Autodesk Inventor part; units mm, degrees
ref_plane "Work Plane1" through (0, 485, 0) normal (0, -1, 0) x (1, 0, 0)
ref_plane "YZ Plane" through (0, 0, 0) normal (1, 0, 0) x (0, 1, 0)
ref_plane "XZ Plane" through (0, 0, 0) normal (0, 1, 0) x (-1, 0, 0)
sketch "Sketch1" plane through (0, 0, 0) normal (0, 1, 0) x (-1, 0, 0)
  line L0 (-12, 14) -> (12, 14) construction
  line L1 (14, 12) -> (14, -12) construction
  line L2 (12, -14) -> (-12, -14) construction
  line L3 (-14, -12) -> (-14, 12) construction
  line L4 (-14, 14) -> (14, -14) construction
  line L5 (14, 14) -> (-14, -14) construction
  arc A0 (14, 12) -> (12, 14) centre (12, 12) ccw construction
  arc A1 (12, -14) -> (14, -12) centre (12, -12) ccw construction
  arc A2 (-14, -12) -> (-12, -14) centre (-12, -12) ccw construction
  arc A3 (-12, 14) -> (-14, 12) centre (-12, 12) ccw construction
  line L6 (-12, -15) -> (12, -15)
  arc A4 (12, -15) -> (15, -12) centre (12, -12) ccw
  line L7 (15, -12) -> (15, 12)
  arc A5 (15, 12) -> (12, 15) centre (12, 12) ccw
  line L8 (12, 15) -> (-12, 15)
  arc A6 (-12, 15) -> (-15, 12) centre (-12, 12) ccw
  line L9 (-15, 12) -> (-15, -12)
  arc A7 (-15, -12) -> (-12, -15) centre (-12, -12) ccw
  line L10 (13, -12) -> (13, 12)
  arc A8 (13, 12) -> (12, 13) centre (12, 12) ccw
  line L11 (12, 13) -> (-12, 13)
  arc A9 (-12, 13) -> (-13, 12) centre (-12, 12) ccw
  line L12 (-13, 12) -> (-13, -12)
  arc A10 (-13, -12) -> (-12, -13) centre (-12, -12) ccw
  line L13 (-12, -13) -> (12, -13)
  arc A11 (12, -13) -> (13, -12) centre (12, -12) ccw
  point P0 (0, 0)
  point P1 (0, 0)
  point P2 (0, 0)
  dimension "d10" = 2
  dimension "depth" = 30
  dimension "width" = 30
  dimension "thickness" = 2
extrude "Extrusion1" add sketch "Sketch1" along normal blind 970
ref_plane "Work Plane1" through (0, 485, 0) normal (0, -1, 0) x (1, 0, 0)
sketch "Sketch3" plane through (12, 0, -15) normal (0, 0, -1) x (-1, 0, 0)
  line L0 (12, -397) -> (12, 2382) construction
  circle A0 centre (-418, 1000) radius 985
  point P0 (12, 0)
  dimension "d29" = 1970
  dimension "d31" = 1000
  dimension "d34" = 430
extrude "Extrusion2" cut sketch "Sketch3" against normal through all keep common part
equation "\"d10\" = thickness"
properties part number "podest duzy profil 3" material "Steel"
Here's how the part is built. I have some questions about the finished solid (model axes, mm). A direction names the side the tool comes from. Give positions to 0.01 mm unless a question says otherwise; leave off trailing zeros. Loops run counter-clockwise (first coordinate to the right, second up) from the corner with the lowest first, then second, coordinate; pieces in that order, holes last. Notation, with made-up numbers: (-13, 27) -> (4, 27) arc R27 cw to (4, 59) -> close; hole circle Ø8 at (45, 50). An arc over 180 degrees is marked (long way). Answer as a JSON object with one key per item and string values. Group by question number.
Item 1: Thinking about a two-plate mould opening in X: for faces 3 (the flat face through (15, 532, 0)), 4 (the flat face through (0, 533, -13)), 5 (the flat face through (14, 970, 0)), which applies, pulls with the +X half, pulls with the -X half, needs draft (parallel to the pull), parting line crosses it, or undercut?
Item 2: Imagine slicing it at B-B on y = 237.5. Write out the boundary of the cut face in (x, z).
Item 3: Imagine slicing it at C-C on x = -3. Write out the boundary of the cut face in (y, z).
Item 4: Will this pin go through, and if not, where does the flat tip stop? pin 1 (10 mm diameter, centred on x = -1, z = -11.5, fed in from -Y).
Item 5: Imagine slicing it at A-A on z = 6.5. Write out the boundary of the cut face in (x, y), then the cut area to 3 significant figures.
Item 6: On a 3-axis mill with a long thin cutter (end or side, diameter ignored), from which of +Z, -Z, +X, -X, +Y, -Y can I reach the whole of each face in a straight line? I mean faces 1 (the flat face through (0, 533, 13)), 2 (the flat face through (0, 533, 15)). Say none if no direction works.
Item 7: I need wall thicknesses on L1, parallel to Z at x = -5, y = 205; L2, parallel to X at y = 463.5, z = -12.5. Which ranges of each line are inside material? Lowest first, please.
Answer list:
{
 "1": {"face 3": "pulls with the +X half", "face 4": "undercut", "face 5": "needs draft"},
 "2": {"outline": "(-15, -12) arc R3 ccw to (-12, -15) -> (12, -15) arc R3 ccw to (15, -12) -> (15, 12) arc R3 ccw to (12, 15) -> (-12, 15) arc R3 ccw to (-15, 12) -> close; hole (-13, -12) arc R1 ccw to (-12, -13) -> (12, -13) arc R1 ccw to (13, -12) -> (13, 12) arc R1 ccw to (12, 13) -> (-12, 13) arc R1 ccw to (-13, 12) -> close"},
 "3": {"outline": "(115.28, -15) -> (970, -15) -> (970, -13) -> (115.28, -13) -> close; (115.28, 13) -> (970, 13) -> (970, 15) -> (115.28, 15) -> close"},
 "4": {"pin 1": "stops at y = 112"},
 "5": {"outline": "(-15, 121.25) arc R985 ccw to (-13, 120.24) -> (-13, 970) -> (-15, 970) -> close; (13, 107.62) arc R985 ccw to (15, 106.69) -> (15, 970) -> (13, 970) -> close", "area": "3,420 mm2"},
 "6": {"face 1": "+Y, -Y", "face 2": "+Z, +X, -X, +Y, -Y"},
 "7": {"L1": "z = -15 to -13, 13 to 15", "L2": "x = -14.96 to -12.87, 12.87 to 14.96"}
}
